```python
from build123d import *

# Parameters (mm, degrees)
PAD002_DEPTH    = 12
POCKET007_DEPTH = 243.567033
POCKET008_DEPTH = 215.317033
SKETCH013_R     = 3.75
PAD003_DEPTH    = 0.5
SKETCH014_R     = 2.75
POCKET009_DEPTH = 77.101
POCKET010_DEPTH = 76.601
POCKET011_DEPTH = 43.551
POCKET012_DEPTH = 43.551


with BuildPart() as part:
    # Sketch010 → Pad002 (new body)
    with BuildSketch(Plane.XY):
        with BuildLine():
            Line((0, 0), (38.05, 0))
            Line((38.05, 0), (38.05, 45.1))
            ThreePointArc((38.05, 45.1), (36.175483, 49.625483), (31.65, 51.5))
            Line((31.65, 51.5), (5, 51.5))
            Line((5, 51.5), (5, 68))
            Line((5, 68), (2.5, 68))
            Line((2.5, 68), (2.5, 54.5))
            Line((2.5, 54.5), (0, 54.5))
            Line((0, 54.5), (0, 0))
        make_face()
    pad002 = extrude(amount=PAD002_DEPTH)

    # Mirrored001: Pad002 across Sketch010 V_Axis
    add(pad002.mirror(Plane(origin=(0, 0, 0), x_dir=(0, 0, 1), z_dir=(1, 0, 0))))

    # Sketch011 (on DatumPlane) → Pocket007 (cut, through all)
    with BuildSketch(Plane.YZ):
        with BuildLine():
            Line((0, 9.8), (58, 9.8))
            ThreePointArc((68, 9.8), (63, 12), (58, 9.8))
            Line((68, 12.8), (68, 9.8))
            Line((0, 12.8), (68, 12.8))
            Line((0, 9.8), (0, 12.8))
        make_face()
    pocket007 = extrude(amount=POCKET007_DEPTH, mode=Mode.SUBTRACT)

    # Mirrored002: Pocket007 across YZ
    add(pocket007.mirror(Plane.YZ), mode=Mode.SUBTRACT)

    # Sketch012 (on DatumPlane) → Pocket008 (cut, through all)
    with BuildSketch(Plane.XY.offset(9.8)):
        Polygon((0, 6.8), (20.35, 6.8), (31.55, 9.6), (31.55, 45.2), (0, 45.2), align=None)
    pocket008 = extrude(amount=-POCKET008_DEPTH, mode=Mode.SUBTRACT)

    # Mirrored003: Pocket008 across Sketch012 V_Axis
    add(pocket008.mirror(Plane(origin=(0, 0, 9.8), x_dir=(0, 0, 1), z_dir=(1, 0, 0))), mode=Mode.SUBTRACT)

    # Sketch013 (on DatumPlane) → Pad003 (join)
    with BuildSketch(Plane.YZ.offset(38.05)):
        with Locations((22.75, 4.9)):
            Circle(SKETCH013_R)
    pad003 = extrude(amount=PAD003_DEPTH)

    # Mirrored004: Pad003 across YZ
    add(pad003.mirror(Plane.YZ))

    # Sketch014 (on DatumPlane) → Pocket009 (cut, through all)
    with BuildSketch(Plane.YZ.offset(38.55)):
        with Locations((22.75, 4.9)):
            Circle(SKETCH014_R)
    extrude(amount=-POCKET009_DEPTH, mode=Mode.SUBTRACT)

    # Sketch015 (on DatumPlane) → Pocket010 (cut, through all)
    with BuildSketch(Plane.YZ.offset(38.05)):
        with BuildLine():
            Line((2, -1), (-1, -1))
            Line((-1, -1), (-1, 10.8))
            Line((-1, 10.8), (2, 10.8))
            Line((2, 10.8), (2, 9.8))
            ThreePointArc((2, 9.8), (0.585786, 9.214214), (0, 7.8))
            Line((0, 7.8), (0, 2))
            ThreePointArc((0, 2), (0.585786, 0.585786), (2, 0))
            Line((2, 0), (2, -1))
        make_face()
    extrude(amount=-POCKET010_DEPTH, mode=Mode.SUBTRACT)

    # Sketch016 (on DatumPlane) → Pocket011 (cut, through all)
    with BuildSketch(Plane.YZ.offset(5)):
        with BuildLine():
            ThreePointArc((66, 0), (67.414214, 0.585786), (68, 2))
            Line((68, 0), (68, 2))
            Line((66, 0), (68, 0))
        make_face()
    extrude(amount=-POCKET011_DEPTH, mode=Mode.SUBTRACT)

    # Sketch017 (on DatumPlane) → Pocket012 (cut, through all)
    with BuildSketch(Plane.YZ.offset(5)):
        with BuildLine():
            ThreePointArc((61.2764, 7.446272), (63, 3.75), (64.7236, 7.446272))
            Line((64.7236, 7.446272), (64.7236, 12.446272))
            Line((61.2764, 12.446272), (64.7236, 12.446272))
            Line((61.2764, 7.446272), (61.2764, 12.446272))
        make_face()
    extrude(amount=-POCKET012_DEPTH, mode=Mode.SUBTRACT)


solid = part.part
```
CAD build for the part. Positions are in the model's coordinates, mm. A direction names the side the tool comes from. Give positions to 0.01 mm unless a question says otherwise; leave off trailing zeros. Write each loop counter-clockwise with the first axis right and the second up, starting at its lowest first coordinate (ties: lowest second). Pieces come first, ordered by that corner, then holes. Notation, with made-up numbers: M -39.75,-8 L 10.25,-8 A28 ccw 10.25,16 Z; hole C 5,46.5 d6. An arc over 180 degrees is marked long. Return JSON: item names as keys, results as strings. Group by question number.
(1) Band-saw the part on C-C (y = 33). Give the cut face in (x, z), and give its area (3 significant figures).
(2) Mould opens along X. For faces 5 (the face through (-38.296, 26.327, 6.026)), 6 (the face through (2.5, 60, 4)), 7 (the face through (0, 54.5, 5)), 8 (the face through (38.55, 22, 8)) say: pulls with the +X half, pulls with the -X half, needs draft (parallel to the pull), parting line crosses it, or undercut.
(3) Band-saw the part on D-D (z = 6.5). State how many separate pieces and enclosed holes the cut face has, and give its area (3 significant figures).
(4) 3-axis set-ups, long thin cutter, end or side, ignore diameter. For faces 1 (the face through (-4, 61.276, 10)), 2 (the face through (0, 45.2, 5)), 3 (the face through (-5, 60, 4)), 4 (the face through (5, 60, 4)): which of +Z, -Z, +X, -X, +Y, -Y reach the whole face in a straight line?
(5) Drill centre lines: L1, parallel to Y at x = 4.35, z = 6; L2, parallel to X at y = 19.5, z = 3.5; L3, parallel to X at y = 26, z = 9. Where is each one in solid material? Low to high. Write a range as [from, to].
(6) Flat gauge pins, fed straight in: pin 1 Ø5 at (y, z) = (50, 5) entering from -X; pin 2 Ø3.5 at (y, z) = (58.5, 7) entering from +X; pin 3 Ø4 at (x, z) = (20, 10) entering from -Y. Where does each tip first touch, or does it go through?
(7) Band-saw the part on A-A (y = 63). Give the cut face in (x, z).
(8) Band-saw the part on B-B (x = 16). Give the cut face in (y, z), and give its area (3 significant figures).
Entries:
{
 "1": {"outline": "M -38.05,0 L -31.55,0 L -31.55,9.8 L -38.05,9.8 Z; M 31.55,0 L 38.05,0 L 38.05,9.8 L 31.55,9.8 Z", "area": "127 mm^2"},
 "2": {"face 5": "needs draft", "face 6": "undercut", "face 7": "undercut", "face 8": "pulls with the +X half"},
 "3": {"separate pieces": "4", "enclosed holes": "0", "area": "1,530 mm^2"},
 "4": {"face 1": "+Z, +X, -X", "face 2": "+Z, -Z", "face 3": "+Z, -Z, -X, +Y", "face 4": "+Z, -Z, +X, +Y"},
 "5": {"L1": "y = [0, 6.8], [45.2, 60.75], [65.25, 68]", "L2": "x = [-38.55, -31.55], [31.55, 38.55]", "L3": "x = [-38.05, -31.55], [31.55, 38.05]"},
 "6": {"pin 1": "stops at x = -37.58", "pin 2": "stops at x = 5", "pin 3": "stops at y = 0.01"},
 "7": {"outline": "M -5,0 L -2.5,0 L -2.5,3.75 L -5,3.75 Z; M 2.5,0 L 5,0 L 5,3.75 L 2.5,3.75 Z"},
 "8": {"outline": "M 0,2 A2 ccw 2,0 L 6.8,0 L 6.8,9.8 L 2,9.8 A2 ccw 0,7.8 Z; M 45.2,0 L 51.5,0 L 51.5,9.8 L 45.2,9.8 Z", "area": "127 mm^2"}
}
